For this review, use the dimensioned drawing (mm, ordinates from the lowest corner) and the shaded views. Round coordinates to 2 decimals unless told otherwise and drop trailing zeros. Write each loop counter-clockwise with the first axis right and the second up, starting at its lowest first coordinate (ties: lowest second). Pieces come first, ordered by that corner, then holes. Notation, with made-up numbers: M 56,20.25 L 93,20.25 A14 ccw 93,29.25 Z; hole C 0.5,48.5 d5. An arc over 180 degrees is marked long. Answer in a Markdown table with one row per item.
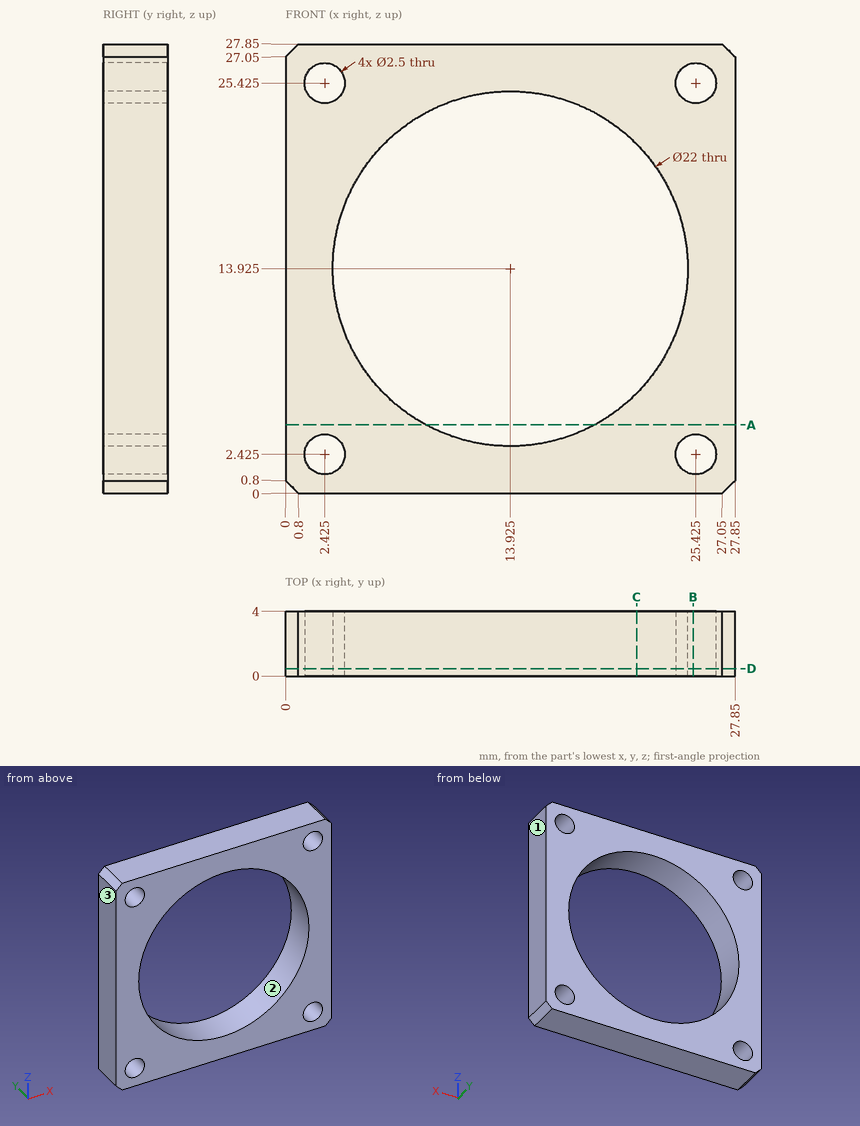
Q1. Mouldability with a two-part tool opening along X and no side actions: class the marked faces 1, 2 and 3 as +X half, -X half, draft (parallel to the pull), parting line (faces both ways), or undercut.
Found:
| item | result |
|---|---|
| face 1 | +X half |
| face 2 | undercut |
| face 3 | -X half |
Q2. Take a section at D-D (y = 0.45). State the section outline as (x, z) points (3 decimals), then the cut area to 3 significant figures.
Found:
| item | result |
|---|---|
| outline | M 0,0.8 L 0.8,0 L 27.05,0 L 27.85,0.8 L 27.85,27.05 L 27.05,27.85 L 0.8,27.85 L 0,27.05 Z; hole C 2.425,2.425 d2.5; hole C 2.425,25.425 d2.5; hole C 13.925,13.925 d22; hole C 25.425,2.425 d2.5; hole C 25.425,25.425 d2.5 |
| area | 375 mm² |
Q3. Take a section at B-B (x = 25.25). State the section outline as (y, z) points.
Found:
| item | result |
|---|---|
| outline | M 0,0 L 4,0 L 4,1.19 L 0,1.19 Z; M 0,3.66 L 4,3.66 L 4,24.19 L 0,24.19 Z; M 0,26.66 L 4,26.66 L 4,27.85 L 0,27.85 Z |
Q4. For probe 1 along Z at (x, y) = (26, 3.75); probe 2 along Z at (x, y) = (14, 3.8); probe 3 along Z at (x, y) = (26.5, 0.8), list the stretches that pass through material, from the lowest coordinate up.
Found:
| item | result |
|---|---|
| probe 1 | 0 to 1.32, 3.53 to 24.32, 26.53 to 27.85 |
| probe 2 | 0 to 2.93, 24.92 to 27.85 |
| probe 3 | 0 to 1.79, 3.06 to 24.79, 26.06 to 27.85 |
Q5. Take a section at C-C (x = 21.75). State the section outline as (y, z) points, then the cut area to 3 significant figures.
Found:
| item | result |
|---|---|
| outline | M 0,0 L 4,0 L 4,6.19 L 0,6.19 Z; M 0,21.66 L 4,21.66 L 4,27.85 L 0,27.85 Z |
| area | 49.6 mm² |
Q6. Take a section at A-A (z = 4.25). State the section outline as (x, y) points, then the cut area to 3 significant figures.
Found:
| item | result |
|---|---|
| outline | M 0,0 L 8.69,0 L 8.69,4 L 0,4 Z; M 19.16,0 L 27.85,0 L 27.85,4 L 19.16,4 Z |
| area | 69.5 mm² |
